CAD build for the part. Positions are in the model's coordinates, mm. A direction names the side the tool comes from. Round coordinates to 2 decimals unless told otherwise and drop trailing zeros. Order: outer loops, then holes, each group sorted by start corner. A loop starts at its lowest first (then second) coordinate and runs counter-clockwise, first axis right, second up.
```python
from build123d import *

# Parameters (mm, degrees)
SKETCH1_R           = 12.7
SKETCH1_R_2         = 10.16
BOSS_EXTRUDE1_DEPTH = 25.4
FILLET1_R           = 1.27
SKETCH2_R           = 15.875
SKETCH2_R_2         = 12.7
BOSS_EXTRUDE2_DEPTH = 3.048
CUT_EXTRUDE1_DEPTH  = 3.048


with BuildPart() as part:
    # Sketch1 → Boss-Extrude1 (new body)
    with BuildSketch(Plane(origin=(0, 0, 0), x_dir=(1, 0, 0), z_dir=(0, 1, 0))):
        with Locations(Location((0, 0, 0), (0, 0, 270))):
            Circle(SKETCH1_R)
        with Locations(Location((0, 0, 0), (0, 0, 270))):
            Circle(SKETCH1_R_2, mode=Mode.SUBTRACT)
    extrude(amount=BOSS_EXTRUDE1_DEPTH)

    # Fillet1
    fillet1_edges = [part.edges().sort_by_distance(p)[0] for p in [
        (0, 25.4, -10.16),
    ]]
    fillet(fillet1_edges, radius=FILLET1_R)

    # Sketch2 → Boss-Extrude2 (add)
    with BuildSketch(Plane.XZ):
        with Locations(Location((0, 0, 0), (0, 0, 270))):
            Circle(SKETCH2_R)
        with Locations(Location((0, 0, 0), (0, 0, 270))):
            Circle(SKETCH2_R_2, mode=Mode.SUBTRACT)
    extrude(amount=-BOSS_EXTRUDE2_DEPTH)

    # Sketch3 → Cut-Extrude1 (cut)
    with BuildSketch(Plane(origin=(0, 3.048, 0), x_dir=(1, 0, 0), z_dir=(0, 1, 0))):
        with BuildLine():
            Line((-1.27, 16.390053577), (-1.27, 12.580053577))
            ThreePointArc((-1.27, 12.580053577), (0, 12.64399652), (1.27, 12.580053577))
            Line((1.27, 12.580053577), (1.27, 16.390053577))
            Line((1.27, 16.390053577), (-1.27, 16.390053577))
        make_face()
        with BuildLine():
            Line((12.580053577, -1.27), (16.390053577, -1.27))
            Line((16.390053577, -1.27), (16.390053577, 1.27))
            Line((16.390053577, 1.27), (12.580053577, 1.27))
            ThreePointArc((12.580053577, 1.27), (12.64399652, 0), (12.580053577, -1.27))
        make_face()
        with BuildLine():
            Line((-1.27, -12.580053577), (-1.27, -16.390053577))
            Line((-1.27, -16.390053577), (1.27, -16.390053577))
            Line((1.27, -16.390053577), (1.27, -12.580053577))
            ThreePointArc((1.27, -12.580053577), (0, -12.64399652), (-1.27, -12.580053577))
        make_face()
        with BuildLine():
            Line((-12.580053577, 1.27), (-16.390053577, 1.27))
            Line((-16.390053577, 1.27), (-16.390053577, -1.27))
            Line((-16.390053577, -1.27), (-12.580053577, -1.27))
            ThreePointArc((-12.580053577, -1.27), (-12.64399652, 0), (-12.580053577, 1.27))
        make_face()
    extrude(amount=-CUT_EXTRUDE1_DEPTH, mode=Mode.SUBTRACT)


solid = part.part
```
1. Tool access for faces 4 (the face through (0.018, 1.545, 12.644)), 5 (the face through (9.1, 3.048, 9.1)), 6 (the face through (-9.1, 3.048, -9.1)): list every direction of +Z, -Z, +X, -X, +Y, -Y with a clear straight run to the whole face (end or side of a thin tool).
2. Drill centre lines: line 1 (X direction, y = 18.25, z = 0); line 2 (Z direction, x = 3.5, y = 17); line 3 (Z direction, x = -3, y = 3). Where is each one in solid material? Low to high.
3. Cut at C-C, the plane y = 17. Write the cut outline in (x, z).
4. Cut at A-A, the plane x = 0. Write the cut outline in (y, z).
5. Pin check, flat tips, straight feed: P1, Ø2.5, axis at x = 13.5, y = 2, coming from the -Z side; P2, Ø12, axis at x = 0, z = 0, coming from the -Y side; P3, Ø6, axis at x = -9, y = 4.5, coming from the -Z side; P4, Ø3.5, axis at x = -14.5, y = 2.5, coming from the +Z side. Stop position of each tip, or through.
6. Cut at B-B, the plane z = 0. Write the cut outline in (x, y), and give its area (3 significant figures).
7. Mould opens along X. For faces 1 (the face through (12.644, 1.545, -0.018)), 2 (the face through (1.27, 2, -14)), 3 (the face through (10, 3.048, -9)) say: released by +X, released by -X, zero draft, split by the parting line, or undercut.
Outcome:
1. face 4: +Z, -Y
1. face 5: +Z, +X, +Y
1. face 6: -Z, -X, +Y
2. line 1: x = -12.7 to -10.16, 10.16 to 12.7
2. line 2: z = -12.21 to -9.54, 9.54 to 12.21
2. line 3: z = -15.59 to -9.71, 9.71 to 15.59
3. outline: circle Ø25.4 at (0, 0); hole circle Ø20.32 at (0, 0)
4. outline: (0, -12.64) - (3.05, -12.64) - (3.05, -12.7) - (25.4, -12.7) - (25.4, -11.43) arc R1.27 ccw to (24.13, -10.16) - (0, -10.16) - close; (0, 10.16) - (24.13, 10.16) arc R1.27 ccw to (25.4, 11.43) - (25.4, 12.7) - (3.05, 12.7) - (3.05, 12.64) - (0, 12.64) - close
5. P1: stops at z = -10.1
5. P2: passes through
5. P3: stops at z = -14.54
5. P4: stops at z = 9.46
6. outline: (-12.7, 3.05) - (-12.64, 3.05) - (-12.64, 0) - (-10.16, 0) - (-10.16, 24.13) arc R1.27 ccw to (-11.43, 25.4) - (-12.7, 25.4) - close; (10.16, 0) - (12.64, 0) - (12.64, 3.05) - (12.7, 3.05) - (12.7, 25.4) - (11.43, 25.4) arc R1.27 ccw to (10.16, 24.13) - close
6. area: 128 mm2
7. face 1: released by +X
7. face 2: undercut
7. face 3: zero draft
